The figure shows three views and two pictorial views of one solid part (mm, origin at its lowest corner). Answer the questions. Round coordinates to 2 decimals unless told otherwise and drop trailing zeros. Write each loop counter-clockwise with the first axis right and the second up, starting at its lowest first coordinate (ties: lowest second). Pieces come first, ordered by that corner, then holes.
Item 1: Find section B-B on y = 74.9. Give the vertices of the cut face in (x, z).
Item 2: Each of these flat-tipped pins is pushed along its axis until it touches: pin 1 (4 mm diameter, centred on x = 117.9, y = 47.16, fed in from +Z); pin 2 (3 mm diameter, centred on x = 7.1, y = 74.9, fed in from -Z); pin 3 (1 mm diameter, centred on x = 55, z = 2.5, fed in from +Y). Where does it stop, or does it pass through?
Item 3: Find section D-D on y = 56. Give the vertices of the cut face in (x, z) (1 decimal).
Item 4: Find section A-A on y = 5.1. Give the vertices of the cut face in (x, z).
Item 5: Find section C-C on x = 92. Give the vertices of the cut face in (y, z).
Item 6: Find the intervals of material crossed by probe 1 along X at (y, z) = (5.1, 0.7); probe 2 along Y at (x, z) = (117.5, 0.5) (1 decimal); probe 3 along Y at (x, z) = (104.5, 1.4), in increasing order.
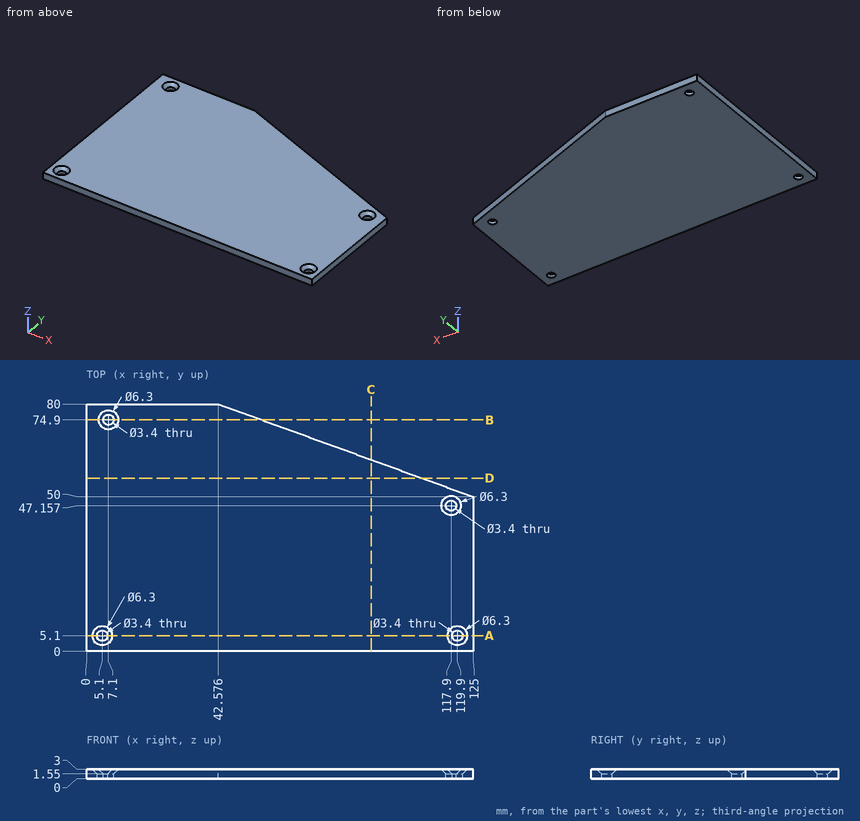
Check values:
1. outline: (0, 0) - (5.4, 0) - (5.4, 1.55) - (3.95, 3) - (0, 3) - close; (8.8, 0) - (56.59, 0) - (56.59, 3) - (10.25, 3) - (8.8, 1.55) - close
2. pin 1: stops at z = 1.85
2. pin 2: passes through
2. pin 3: stops at y = 75.66
3. outline: (0, 0) - (108.5, 0) - (108.5, 3) - (0, 3) - close
4. outline: (0, 0) - (3.4, 0) - (3.4, 1.55) - (1.95, 3) - (0, 3) - close; (6.8, 0) - (118.2, 0) - (118.2, 1.55) - (116.75, 3) - (8.25, 3) - (6.8, 1.55) - close; (121.6, 0) - (125, 0) - (125, 3) - (123.05, 3) - (121.6, 1.55) - close
5. outline: (0, 0) - (62.01, 0) - (62.01, 3) - (0, 3) - close
6. probe 1: x = 0 to 3.4, 6.8 to 118.2, 121.6 to 125
6. probe 2: y = 0 to 45.5, 48.8 to 52.7
6. probe 3: y = 0 to 57.46
